Work out the finished part from the listing and answer in its coordinate system (mm). A direction names the side the tool comes from. Give positions to 0.01 mm unless a question says otherwise; leave off trailing zeros. Order: outer loops, then holes, each group sorted by start corner. A loop starts at its lowest first (then second) coordinate and runs counter-clockwise, first axis right, second up.
```python
from build123d import *

# Parameters (mm, degrees)
SKETCH1_W           = 40
SKETCH1_H           = 33.6
BOSS_EXTRUDE1_DEPTH = 20
SKETCH2_W           = 7.1
SKETCH2_H           = 2.4
BOSS_EXTRUDE2_DEPTH = 20
SKETCH4_R           = 2.2
CUT_EXTRUDE1_DEPTH  = 3
BOSS_EXTRUDE4_DEPTH = 1.8
SKETCH6_R           = 1.5
CUT_EXTRUDE2_DEPTH  = 1.2
SKETCH7_R           = 6
BOSS_EXTRUDE5_DEPTH = 1.2
SKETCH8_R           = 5.5
BOSS_EXTRUDE6_DEPTH = 0.8
SKETCH10_R          = 2.5
BOSS_EXTRUDE8_DEPTH = 3.8
BOSS_EXTRUDE9_DEPTH = 4
CIRPATTERN2_COUNT   = 30
SKETCH12_R          = 1.5
CUT_EXTRUDE4_DEPTH  = 4


with BuildPart() as part:
    # Sketch1 → Boss-Extrude1 (new body)
    with BuildSketch(Plane.XY):
        with Locations((-4.683412042, -8.529571984)):
            Rectangle(SKETCH1_W, SKETCH1_H)
    extrude(amount=BOSS_EXTRUDE1_DEPTH)

    # Sketch2 → Boss-Extrude2 (add)
    with BuildSketch(Plane.XY.offset(20)):
        with Locations((18.866587958, 0.270428016)):
            Rectangle(SKETCH2_W, SKETCH2_H)
        with Locations((-28.233412042, 0.270428016)):
            Rectangle(SKETCH2_W, SKETCH2_H)
    extrude(amount=-BOSS_EXTRUDE2_DEPTH)

    # Sketch4 → Cut-Extrude1 (cut)
    with BuildSketch(Plane(origin=(0, 1.470428016, 0), x_dir=(1, 0, 0), z_dir=(0, 1, 0))):
        with Locations((19.066587958, -15)):
            Circle(SKETCH4_R)
        with Locations((19.066587958, -5)):
            Circle(SKETCH4_R)
        with Locations((-28.433412042, -15)):
            Circle(SKETCH4_R)
        with Locations((-28.433412042, -5)):
            Circle(SKETCH4_R)
    extrude(amount=-CUT_EXTRUDE1_DEPTH, mode=Mode.SUBTRACT)

    # Sketch5 → Boss-Extrude4 (add)
    with BuildSketch(Plane(origin=(0, 8.270428016, 0), x_dir=(1, 0, 0), z_dir=(0, 1, 0))):
        with BuildLine():
            Line((-15.433412042, -0.2), (-15.433412042, -19.8))
            Line((-15.433412042, -19.8), (4.566587958, -19.8))
            ThreePointArc((4.566587958, -19.8), (15.11483144, -10), (4.566587958, -0.2))
            Line((4.566587958, -0.2), (-15.433412042, -0.2))
        make_face()
    extrude(amount=BOSS_EXTRUDE4_DEPTH)

    # Sketch6 → Cut-Extrude2 (cut)
    with BuildSketch(Plane.XZ.offset(25.329571984)):
        with Locations((-22.660585011, 17.329722527)):
            Circle(SKETCH6_R)
        with Locations((-22.660585011, 1.487126069)):
            Circle(SKETCH6_R)
        with Locations((14.670467636, 17.329722527)):
            Circle(SKETCH6_R)
        with Locations((14.670467636, 1.487126069)):
            Circle(SKETCH6_R)
    extrude(amount=-CUT_EXTRUDE2_DEPTH, mode=Mode.SUBTRACT)

    # Sketch7 → Boss-Extrude5 (add)
    with BuildSketch(Plane(origin=(0, 10.070428016, 0), x_dir=(1, 0, 0), z_dir=(0, 1, 0))):
        with Locations((5.288292978, -10)):
            Circle(SKETCH7_R)
    extrude(amount=BOSS_EXTRUDE5_DEPTH)

    # Sketch8 → Boss-Extrude6 (add)
    with BuildSketch(Plane(origin=(0, 11.270428016, 0), x_dir=(1, 0, 0), z_dir=(0, 1, 0))):
        with Locations((5.316587958, -10)):
            Circle(SKETCH8_R)
    extrude(amount=BOSS_EXTRUDE6_DEPTH)

    # Sketch10 → Boss-Extrude8 (add)
    with BuildSketch(Plane(origin=(0, 12.070428016, 0), x_dir=(1, 0, 0), z_dir=(0, 1, 0))):
        with Locations((5.316587958, -10)):
            Circle(SKETCH10_R)
    extrude(amount=BOSS_EXTRUDE8_DEPTH)

    # Sketch11 → Boss-Extrude9 (add)
    with BuildSketch(Plane(origin=(0, 15.870428016, 0), x_dir=(1, 0, 0), z_dir=(0, 1, 0))):
        Polygon((5.503448723, -6.801928291), (5.271899273, -7.500399448), (5.664716985, -7.524357421), align=None)
    boss_extrude9 = extrude(amount=-BOSS_EXTRUDE9_DEPTH)

    # CirPattern2: Boss-Extrude9 ×30 about axis
    cirpattern2_axis = Axis((5.316587958, 0, 10), (0, 1, 0))
    for i in range(1, CIRPATTERN2_COUNT):
        add(boss_extrude9.rotate(cirpattern2_axis, i * 360 / CIRPATTERN2_COUNT))

    # Sketch12 → Cut-Extrude4 (cut)
    with BuildSketch(Plane(origin=(0, 15.870428016, 0), x_dir=(1, 0, 0), z_dir=(0, 1, 0))):
        with Locations((5.316587958, -10)):
            Circle(SKETCH12_R)
    extrude(amount=-CUT_EXTRUDE4_DEPTH, mode=Mode.SUBTRACT)


solid = part.part
```
1. Given P1, Ø0.9, axis at x = -22.5, z = 1.5, coming from the -Y side; P2, Ø6, axis at x = -5, z = 10, coming from the +Y side; P3, Ø2.5, axis at x = -22.66, z = 17.33, coming from the +Y side; P4, Ø4, axis at x = 19.07, z = 5, coming from the +Y side, each flat-ended and moving along its own axis, determine where each tip first touches the part or whether it passes through.
Findings below:
P1: stops at y = -24.13
P2: stops at y = 10.07
P3: stops at y = 8.27
P4: passes through
2. The part is cut by section C-C (x = -10). Write down the section's boundary in (y, z), then the cut area to 3 significant figures.
Findings below:
outline: (-25.33, 0) - (8.27, 0) - (8.27, 0.2) - (10.07, 0.2) - (10.07, 19.8) - (8.27, 19.8) - (8.27, 20) - (-25.33, 20) - close
area: 707 mm2
3. Straight lines are drawn through the part: probe 1 along X at (y, z) = (0.1, 5); probe 2 along X at (y, z) = (0, 14.25); probe 3 along Y at (x, z) = (-7, 4.25). For each, find the intervals that lie inside material, in ascending order.
Findings below:
probe 1: x = -31.78 to -30.63, -26.23 to 16.87, 21.27 to 22.42
probe 2: x = -31.78 to -30.5, -26.37 to 17, 21.13 to 22.42
probe 3: y = -25.33 to 10.07
4. The part is cut by section B-B (z = 6). State how many separate pieces and enclosed holes the cut face has, then the cut area to 3 significant figures.
Findings below:
separate pieces: 3
enclosed holes: 0
area: 1,430 mm2
5. Which of the six approach directions +Z, -Z, +X, -X, +Y, -Y give full straight-line access (tool end or side, diameter ignored) to faces 5 (the face through (-24.683, -13, 10)), 6 (the face through (15.317, -13, 10)), 7 (the face through (4.12, 11.66, 15.37))?
Findings below:
face 5: +Z, -Z, -X, -Y
face 6: +Z, -Z, +X, -Y
face 7: +Y
6. The mould has two halves that part along Z. Classify faces 1 (the face through (-5, -8, 0)), 2 (the face through (21.1, 0.29, 15.84)), 3 (the face through (-26.4, 0.29, 5.84)), 4 (the face through (-17, 8.27, 11)): pulls with the +Z half, pulls with the -Z half, needs draft (parallel to the pull), parting line crosses it, or undercut.
Findings below:
face 1: pulls with the -Z half
face 2: undercut
face 3: undercut
face 4: needs draft
7. The part is cut by section A-A (x = 18). Write down the section's boundary in (y, z).
Findings below:
outline: (-0.93, 0) - (1.47, 0) - (1.47, 3.08) - (-0.93, 3.08) - close; (-0.93, 6.92) - (1.47, 6.92) - (1.47, 13.08) - (-0.93, 13.08) - close; (-0.93, 16.92) - (1.47, 16.92) - (1.47, 20) - (-0.93, 20) - close
8. The part is cut by section D-D (y = -2). Write down the section's boundary in (x, z), then the cut area to 3 significant figures.
Findings below:
outline: (-24.68, 0) - (15.32, 0) - (15.32, 20) - (-24.68, 20) - close
area: 800 mm2
